Autodesk Fusion 360 part; units mm, degrees
sketch "Esquisse1" plane through (0, 0, 0) normal (0, 0, 1) x (1, 0, 0)
  circle A0 centre (0, 0) radius 7.5
  dimension "d1" = 15
extrude "Extrusion1" add sketch "Esquisse1" along normal blind 5
sketch "Esquisse2" plane through (0, 0, 0) normal (0, 1, 0) x (1, 0, 0)
sketch "Esquisse3" plane through (0, 0, 0) normal (0, 1, 0) x (1, 0, 0)
  line L0 (3, -3.5) -> (8.18, -4.4134)
  line L1 (8.18, -4.4134) -> (8.18, -0.5866)
  line L2 (8.18, -0.5866) -> (3, -1.5)
  line L3 (3, -1.5) -> (3, -3.5)
  line L4 (0, -1.75) -> (0, -22.5)
  dimension "d4" = 2
  dimension "d6" = 1.5
  dimension "d7" = 100
  dimension "d8" = 100
  dimension "d9" = 3
revolve "Révolution1" cut sketch "Esquisse3" angle 360 about axis through (0, 0, 1.75) along (0, 0, 1)
sketch "Esquisse4" plane through (0, 0, 5) normal (0, 0, 1) x (-1, 0, 0)
  circle A0 centre (0, 0) radius 7.5
  circle A1 centre (0, 0) radius 6
  dimension "d11" = 12
extrude "Extrusion2" add sketch "Esquisse4" along normal blind 8 contours A1
sketch "Esquisse5" plane through (0, 0, 13) normal (0, 0, 1) x (-1, 0, 0)
  circle A0 centre (0, 0) radius 6
  circle A1 centre (0, 0) radius 2.625
  dimension "d14" = 5.25
sketch "Esquisse6" plane through (0, 0, 13) normal (0, 0, 1) x (1, 0, 0)
extrude "Extrusion3" cut sketch "Esquisse5" against normal blind 7 contours A1
sketch "Esquisse7" plane through (0, 0, 0) normal (0, 1, 0) x (1, 0, 0)
  circle A0 centre (0, -10) radius 1.35
  line L0 (-6, -13) -> (6, -13)
  dimension "d17" = 2.7
  dimension "d18" = 3
extrude "Extrusion4" cut sketch "Esquisse7" along normal blind 15.5
Design review of the part built by this model. Coordinates are the model's own, in mm. A direction names the side the tool comes from. Coordinates: 2 decimals unless noted, no trailing zeros. Loops run counter-clockwise (first coordinate to the right, second up) from the corner with the lowest first, then second, coordinate; pieces in that order, holes last. Notation, with made-up numbers: (15.5, -17) -> (24.5, -17) arc R16 ccw to (24.5, -6) -> close; hole circle Ø2 at (-27.5, -10). An arc over 180 degrees is marked (long way). Answer as a JSON object with one key per item and string values.
Q1. Take a section at C-C on z = 8. Give the boundary of the cut face in (x, y) (3 decimals).
Answer block:
{"outline": "circle Ø12 at (0, 0); hole circle Ø5.25 at (0, 0)"}
Q2. Tool access review of faces 4 (the cylindrical face through (0.342, -2.603, 9.549)), 5 (the cylindrical face through (-7.493, -0.33, 0.348)), 6 (the cylindrical face through (-1.35, 4.1, 10.06)), 7 (the cylindrical face through (-3, 0, 3)), 8 (the flat face through (-3, 1, 13)): name each direction out of +Z, -Z, +X, -X, +Y, -Y from which nothing blocks a thin tool from reaching the whole face with its end or side.
Answer block:
{"face 4": "+Z", "face 5": "+Z, -Z", "face 6": "+Y", "face 7": "none", "face 8": "+Z, +X, -X, +Y, -Y"}
Q3. Clearance check with flat-ended pins moving along their axes: pin 1 Ø3 at (x, y) = (0, 0) entering from -Z; pin 2 Ø6 at (x, z) = (-5.5, 3.5) entering from +Y; pin 3 Ø1.5 at (x, z) = (-2.5, 4) entering from -Y; pin 4 Ø4 at (y, z) = (-4, 9.5) entering from -X. State where each tip first meets the part, or that it passes through.
Answer block:
{"pin 1": "stops at z = 0", "pin 2": "stops at y = 7.03", "pin 3": "stops at y = -7.28", "pin 4": "stops at x = -5.66"}
Q4. Take a section at B-B on y = 0. Give the boundary of the cut face in (x, z) (1 decimal), plus the area to 3 significant figures.
Answer block:
{"outline": "(-7.5, 0) -> (7.5, 0) -> (7.5, 0.7) -> (3, 1.5) -> (3, 3.5) -> (7.5, 4.3) -> (7.5, 5) -> (6, 5) -> (6, 13) -> (2.6, 13) -> (2.6, 6) -> (-2.6, 6) -> (-2.6, 13) -> (-6, 13) -> (-6, 5) -> (-7.5, 5) -> (-7.5, 4.3) -> (-3, 3.5) -> (-3, 1.5) -> (-7.5, 0.7) -> close", "area": "109 mm^2"}
Q5. The part is to be moulded in two halves that separate along Y. For faces 1 (the flat face through (0, 0, 0)), 2 (the flat face through (0, 0, 6)), 3 (the cylindrical face through (1.301, -5.857, 8.944)), say which applies: +Y half, -Y half, draft (parallel to the pull), parting line (faces both ways), or undercut.
Answer block:
{"face 1": "draft", "face 2": "undercut", "face 3": "parting line"}
Q6. To check wall thickness, follow L1, parallel to Z at x = 0, y = 4.9; L2, parallel to Z at x = 0, y = 4.35; L3, parallel to Y at x = 0, z = 8 (3 decimals). State the ranges of each line that lie inside material, in increasing order.
Answer block:
{"L1": "z = 0 to 1.16, 3.84 to 8.65, 11.35 to 13", "L2": "z = 0 to 1.26, 3.74 to 8.65, 11.35 to 13", "L3": "y = -6 to -2.625, 2.625 to 6"}
Q7. Take a section at D-D on y = 5. Give the number of separate pieces and of enclosed holes in the cut face, plus the area to 3 significant figures.
Answer block:
{"separate pieces": "2", "enclosed holes": "1", "area": "69.4 mm^2"}
